Answer from the drawing. Dimensions are ordinates in mm from the lowest x, y and z of the part. A direction names the side the tool comes from. Give positions to 0.01 mm unless a question says otherwise; leave off trailing zeros. Loops run counter-clockwise (first coordinate to the right, second up) from the corner with the lowest first, then second, coordinate; pieces in that order, holes last. Notation, with made-up numbers: (-24.5, -38) -> (34.5, -38) arc R15 cw to (34.5, -14) -> close; hole circle Ø4 at (7.25, -34). An arc over 180 degrees is marked (long way). Write each question's results on one line, items separated by ' | '. Start each with the question number.
Item 1: Determine the mould class of the marked faces 4, 5 and 6 for opening direction X: +X half, -X half, draft (parallel to the pull), parting line (faces both ways), or undercut.
Item 2: Section B-B on x = 8.75 is taken. Write down the section's boundary in (y, z).
Item 3: Section C-C on y = 4 is taken. Write down the section's boundary in (x, z), and give its area (3 significant figures).
Item 4: Which of the six approach directions +Z, -Z, +X, -X, +Y, -Y give full straight-line access (tool end or side, diameter ignored) to the marked faces 1, 2 and 3?
Item 5: This flat-tipped pin is pushed along its axis until it touches: P1, Ø2, axis at y = 35.5, z = 12.5, coming from the +X side. Where does it stop, or does it pass through?
Item 6: Section A-A on z = 7.5 is taken. Write down the section's boundary in (x, y).
Item 7: Section D-D on x = 1.25 is taken. Write down the section's boundary in (y, z).
Item 8: Find the intervals of material crossed by line 1 (Y direction, x = 8.25, z = 10.25); line 2 (Z direction, x = 2.25, y = 29); line 3 (Y direction, x = 3, z = 11), in increasing order.
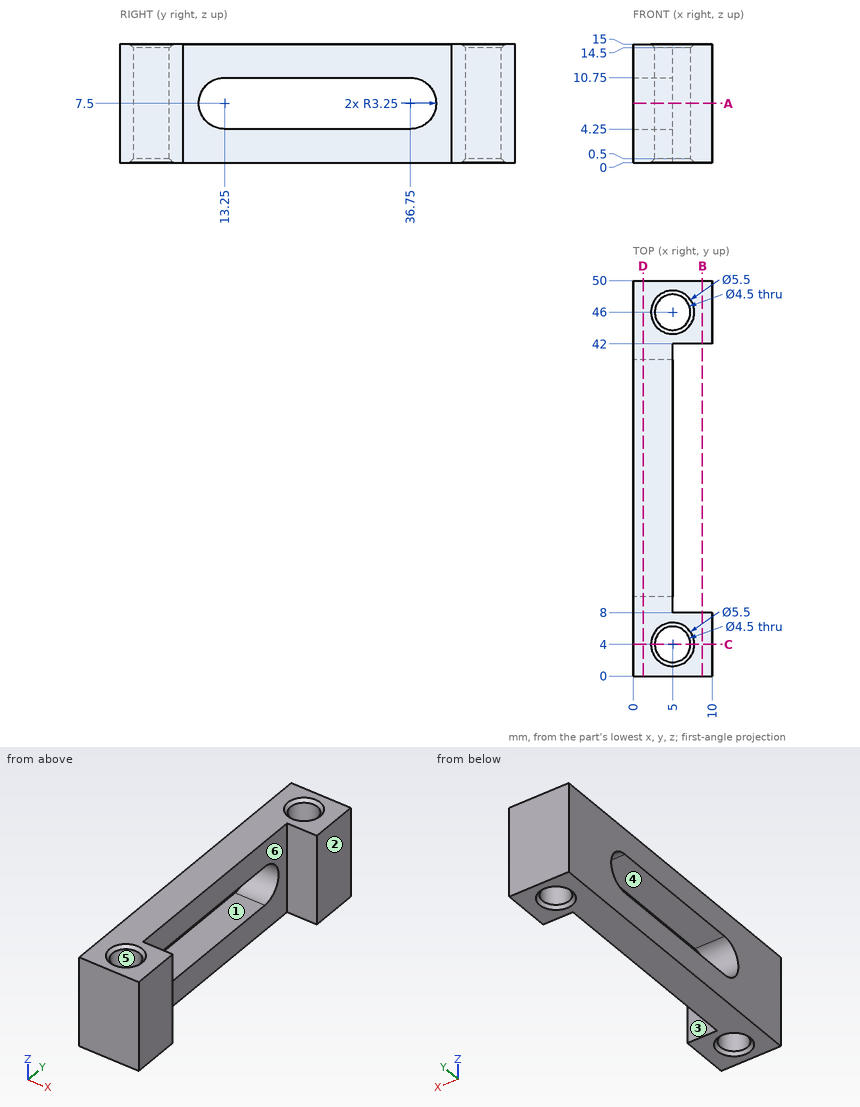
Findings:
1) face 4: draft | face 5: undercut | face 6: +X half
2) outline: (0, 0) -> (8, 0) -> (8, 15) -> (0, 15) -> close; (42, 0) -> (50, 0) -> (50, 15) -> (42, 15) -> close
3) outline: (0, 0) -> (2.25, 0) -> (2.75, 0.5) -> (2.75, 14.5) -> (2.25, 15) -> (0, 15) -> close; (7.25, 0.5) -> (7.75, 0) -> (10, 0) -> (10, 15) -> (7.75, 15) -> (7.25, 14.5) -> close | area: 82.0 mm2
4) face 1: +X, -X | face 2: +Z, -Z, +X, +Y, -Y | face 3: +Z, -Z, +X
5) P1: x = 5
6) outline: (0, 0) -> (10, 0) -> (10, 8) -> (5, 8) -> (5, 10) -> (0, 10) -> close; (0, 40) -> (5, 40) -> (5, 42) -> (10, 42) -> (10, 50) -> (0, 50) -> close; hole circle Ø4.5 at (5, 4); hole circle Ø4.5 at (5, 46)
7) outline: (0, 0) -> (50, 0) -> (50, 15) -> (0, 15) -> close; hole (13.25, 4.25) -> (36.75, 4.25) arc R3.25 ccw to (36.75, 10.75) -> (13.25, 10.75) arc R3.25 ccw to start
8) line 1: 0 to 8, 42 to 50 | line 2: 0 to 4.25, 10.75 to 15 | line 3: 0 to 2.97, 5.03 to 44.97, 47.03 to 50
